Input: part model. Units: mm. Frame: model coordinates. Face numbers are marked on the shaded views. A direction names the side the tool comes from. Coordinates: 2 decimals unless noted, no trailing zeros. Order: outer loops, then holes, each group sorted by start corner. A loop starts at its lowest first (then second) coordinate and runs counter-clockwise, first axis right, second up. Notation, with made-up numbers: M 60.5,-10.5 L 84.5,-10.5 A13 ccw 84.5,6.5 Z; hole C 84,89 d1. An arc over 180 degrees is marked long. One line per item, written item: value.
```python
from build123d import *

# Parameters (mm, degrees)
SKETCH5_R          = 1.15
SKETCH5_R_2        = 0.749999784
BASE_EXTRUDE_DEPTH = 14.000000432
SKETCH9_OUTSIDE_W  = 24.639
SKETCH9_OUTSIDE_H  = 20.632
CUT_EXTRUDE2_DEPTH = 37.000000432


with BuildPart() as part:
    # Sketch5 → Base-Extrude (new body)
    with BuildSketch(Plane.XY):
        with BuildLine():
            Line((-14.650000216, 1.992481203), (-2.16e-07, 2.000000047))
            ThreePointArc((-2.16e-07, 2.000000047), (2.000000047, 1.08e-07), (0, -2.000000047))
            Line((0, -2.000000047), (-15.999999829, -2.000000047))
            Line((-15.999999829, -2.000000047), (-15.999999829, 0.500000071))
            ThreePointArc((-15.999999829, 0.500000071), (-15.656001468, 1.545642629), (-14.650000216, 1.992481203))
        make_face()
        with Locations((-13.500000216, 4.7e-08)):
            Circle(SKETCH5_R, mode=Mode.SUBTRACT)
        Circle(SKETCH5_R_2, mode=Mode.SUBTRACT)
    extrude(amount=-BASE_EXTRUDE_DEPTH)

    # Sketch9 outside → Cut-Extrude2 (cut)
    with BuildSketch(Plane(origin=(0, 17.539650086, 0), x_dir=(-1, 0, 0), z_dir=(0, 1, 0))):
        with Locations((7.0035, -7)):
            Rectangle(SKETCH9_OUTSIDE_W, SKETCH9_OUTSIDE_H)
        Polygon((5.500000203, -12.500000186), (15.999999829, -12.500000186), (15.999999829, -14.000000432), (-1.999999397, -14.000000432), (-1.999999397, -12.500000186), (0, -12.500000186), (0, -1.500000246), (-1.999999397, -1.500000246), (-1.999999397, 0), (15.999999829, 0), (15.999999829, -1.500000246), (5.500000203, -1.500000246), (1.000000164, -1.500000246), (1.000000164, -12.500000186), align=None, mode=Mode.SUBTRACT)
    extrude(amount=-CUT_EXTRUDE2_DEPTH, mode=Mode.SUBTRACT)


solid = part.part
```
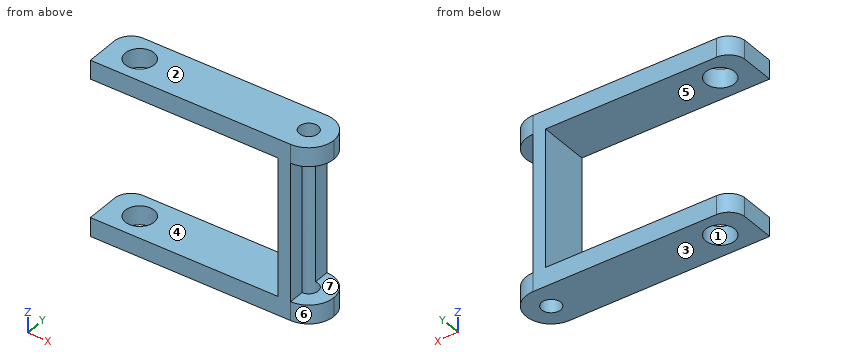
(1) Ray query, line 1 (Z direction, x = -1.5, y = 1.3); line 2 (Y direction, x = -13.5, z = -0.9); line 3 (X direction, y = -1.3, z = -2.5). Return the intervals inside material, ascending. Write a range as from..to.
Data:
line 1: z = -14..-12.5, -1.5..0
line 2: y = -2..-1.15, 1.15..1.99
line 3: x = -1..0
(2) Draft query along Z for the marked faces 1, 2, 3 and 4. Return one class per face: released by +Z, released by -Z, zero draft, split by the parting line, or undercut.
Data:
face 1: zero draft
face 2: released by +Z
face 3: released by -Z
face 4: undercut
(3) Access query for the marked faces 5, 6 and 7. Directions: +Z, -Z, +X, -X, +Y, -Y. A direction counts if a zero-diameter tool reaches every point of the face in a straight line with its end or side. Return the directions, or none.
Data:
face 5: -X, +Y, -Y
face 6: +Z, -Z, +X, -Y
face 7: +X, +Y, -Y
(4) Cut plane B-B on y = -0.25. Output: boundary loops of the cut face in (x, z), plus the area to 3 significant figures.
Data:
outline: M -16,-14 L -14.62,-14 L -14.62,-12.5 L -16,-12.5 Z; M -16,-1.5 L -14.62,-1.5 L -14.62,0 L -16,0 Z; M -12.38,-14 L -0.71,-14 L -0.71,0 L -12.38,0 L -12.38,-1.5 L -1,-1.5 L -1,-12.5 L -12.38,-12.5 Z; M 0.71,-14 L 1.98,-14 L 1.98,-12.5 L 0.71,-12.5 Z; M 0.71,-1.5 L 1.98,-1.5 L 1.98,0 L 0.71,0 Z
area: 46.2 mm2
(5) Cut plane A-A on x = -8.5. Output: boundary loops of the cut face in (y, z), plus the area to 3 significant figures.
Data:
outline: M -2,-14 L 2,-14 L 2,-12.5 L -2,-12.5 Z; M -2,-1.5 L 2,-1.5 L 2,0 L -2,0 Z
area: 12.0 mm2
(6) Cut plane D-D on y = -1.5. Output: boundary loops of the cut face in (x, z).
Data:
outline: M -16,-14 L 1.32,-14 L 1.32,-12.5 L 0,-12.5 L 0,-1.5 L 1.32,-1.5 L 1.32,0 L -16,0 L -16,-1.5 L -1,-1.5 L -1,-12.5 L -16,-12.5 Z
(7) First-contact query: pin 1 (2 mm diameter, centred on y = 1.5, z = -10.5, fed in from +X); pin 2 (1.5 mm diameter, centred on y = 1.5, z = -12.5, fed in from +X); pin 3 (2 mm diameter, centred on y = -1, z = -6.5, fed in from -X). Flat tips, straight axial feed; report the tip coordinate or a pass-through.
Data:
pin 1: stops at x = 0
pin 2: stops at x = 1.85
pin 3: stops at x = -1
(8) Cut plane C-C on x = -13.5. Output: boundary loops of the cut face in (y, z).
Data:
outline: M -2,-14 L -1.15,-14 L -1.15,-12.5 L -2,-12.5 Z; M -2,-1.5 L -1.15,-1.5 L -1.15,0 L -2,0 Z; M 1.15,-14 L 1.99,-14 L 1.99,-12.5 L 1.15,-12.5 Z; M 1.15,-1.5 L 1.99,-1.5 L 1.99,0 L 1.15,0 Z
